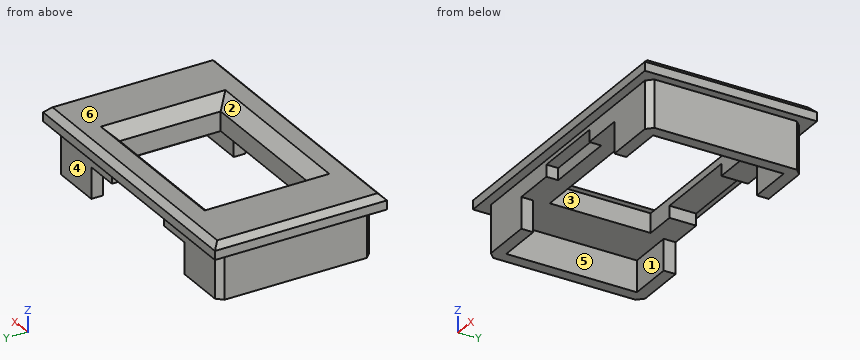
from build123d import *

# Parameters (mm, degrees)
SKETCH_W        = 45
SKETCH_H        = 26
PAD_DEPTH       = 8
SKETCH001_W     = 48
SKETCH001_H     = 29
PAD001_DEPTH    = 2.5
SKETCH002_W     = 25
SKETCH002_H     = 17
POCKET_DEPTH    = 10.501
SKETCH003_W     = 41
SKETCH003_H     = 22
POCKET001_DEPTH = 5.25
SKETCH004_W     = 26
SKETCH004_H     = 27.5
POCKET002_DEPTH = 5.251
SKETCH005_W     = 12
SKETCH005_H     = 2.5
POCKET003_DEPTH = 2
SKETCH006_W     = 14.5
SKETCH006_H     = 4.5
POCKET004_DEPTH = 2
CHAMFER_SIZE    = 1
CHAMFER001_SIZE = 2
CHAMFER002_SIZE = 1


with BuildPart() as part:
    # Sketch → Pad (new body)
    with BuildSketch(Plane.XY):
        Rectangle(SKETCH_W, SKETCH_H)
    extrude(amount=PAD_DEPTH)

    # Sketch001 (on Face6 of Pad) → Pad001 (join)
    with BuildSketch(Plane.XY.offset(8)):
        Rectangle(SKETCH001_W, SKETCH001_H)
    extrude(amount=PAD001_DEPTH)

    # Sketch002 (on Face5 of Pad001) → Pocket (cut, through all)
    with BuildSketch(Plane.XY.offset(10.5)):
        Rectangle(SKETCH002_W, SKETCH002_H)
    extrude(amount=-POCKET_DEPTH, mode=Mode.SUBTRACT)

    # Sketch003 (on Face15 of Pocket) → Pocket001 (cut)
    with BuildSketch(Plane(origin=(0, 0, 0), x_dir=(1, 0, 0), z_dir=(0, 0, -1))):
        Rectangle(SKETCH003_W, SKETCH003_H)
    extrude(amount=-POCKET001_DEPTH, mode=Mode.SUBTRACT)

    # Sketch004 (on Face16 of Pocket001) → Pocket002 (cut, through all)
    with BuildSketch(Plane(origin=(0, 0, 5.25), x_dir=(1, 0, 0), z_dir=(0, 0, -1))):
        Rectangle(SKETCH004_W, SKETCH004_H)
    extrude(amount=POCKET002_DEPTH, mode=Mode.SUBTRACT)

    # Sketch005 (on Face17 of Pocket002) → Pocket003 (cut)
    with BuildSketch(Plane(origin=(0, 0, 5.25), x_dir=(1, 0, 0), z_dir=(0, 0, -1))):
        with Locations((0, 12.25)):
            Rectangle(SKETCH005_W, SKETCH005_H)
    extrude(amount=-POCKET003_DEPTH, mode=Mode.SUBTRACT)

    # Sketch006 (on Face27 of Pocket003) → Pocket004 (cut)
    with BuildSketch(Plane(origin=(0, 0, 5.25), x_dir=(1, 0, 0), z_dir=(0, 0, -1))):
        with Locations((0, -10.75)):
            Rectangle(SKETCH006_W, SKETCH006_H)
    extrude(amount=-POCKET004_DEPTH, mode=Mode.SUBTRACT)

    # Chamfer
    chamfer_edges = [part.edges().sort_by_distance(p)[0] for p in [
        (24, 0, 10.5),
        (0, -14.5, 10.5),
        (0, 14.5, 10.5),
        (-24, 0, 10.5),
    ]]
    chamfer(chamfer_edges, length=CHAMFER_SIZE)

    # Chamfer001
    chamfer001_edges = [part.edges().sort_by_distance(p)[0] for p in [
        (0, 8.5, 10.5),
        (-12.5, 0, 10.5),
        (0, -8.5, 10.5),
        (12.5, 0, 10.5),
    ]]
    chamfer(chamfer001_edges, length=CHAMFER001_SIZE)

    # Chamfer002
    chamfer002_edges = [part.edges().sort_by_distance(p)[0] for p in [
        (-22.5, 13, 4),
        (-22.5, -13, 4),
        (22.5, 13, 4),
        (22.5, -13, 4),
    ]]
    chamfer(chamfer002_edges, length=CHAMFER002_SIZE)


solid = part.part
The model under review builds one solid part; all positions refer to its coordinate system, in mm. Face numbers are marked on the shaded views. A direction names the side the tool comes from. Round coordinates to 2 decimals unless told otherwise and drop trailing zeros. Write each loop counter-clockwise with the first axis right and the second up, starting at its lowest first coordinate (ties: lowest second). Pieces come first, ordered by that corner, then holes. Notation, with made-up numbers: (23, 31.25) - (37, 31.25) arc R10 ccw to (37, 48.25) - close; hole circle Ø6 at (83.5, 1.25). An arc over 180 degrees is marked (long way). One line per item, written item: value. Start each with the question number.
1. Consider section C-C on y = 7. Write out the cut boundary in (x, z), and give its area (4 significant figures).
2. Consider section B-B on x = -2. Write out the cut boundary in (y, z), and give its area (4 significant figures).
3. To check wall thickness, follow L1, parallel to X at y = 5.5, z = 5; L2, parallel to X at y = 3.5, z = 9; L3, parallel to Y at x = 8, z = 7. State the ranges of each line that lie inside material, in increasing order. Write a range as from..to.
4. Clearance check with flat-ended pins moving along their axes: P1, Ø1, axis at y = 11, z = 6.5, coming from the +X side; P2, Ø4, axis at x = 18.5, z = 1.5, coming from the -Y side; P3, Ø1.6, axis at x = -4.5, z = 6.5, coming from the +Y side; P4, Ø6, axis at x = 11, y = 9, coming from the -Z side. State where each tip first meets the part, or that it passes through.
5. Consider section A-A on z = 2.75. Write out the cut boundary in (x, y), and give its area (3 significant figures).
6. The part is to be moulded in two halves that separate along Y. For the marked faces 4, 5 and 6, say which applies: released by +Y, released by -Y, zero draft, split by the parting line, or undercut.
7. Consider section D-D on z = 9. Write out the cut boundary in (x, y), and give its area (3 significant figures).
8. Machinability: for the marked faces 1, 2 and 3, which of the approach directions +Z, -Z, +X, -X, +Y, -Y give a long, thin tool a straight path to every point of the face, cutting with its end or side? Answer none if there is none.
Checks:
1. outline: (-24, 8) - (-22.5, 8) - (-22.5, 0) - (-20.5, 0) - (-20.5, 5.25) - (-12.5, 5.25) - (-12.5, 8.5) - (-14.5, 10.5) - (-23, 10.5) - (-24, 9.5) - close; (12.5, 5.25) - (20.5, 5.25) - (20.5, 0) - (22.5, 0) - (22.5, 8) - (24, 8) - (24, 9.5) - (23, 10.5) - (14.5, 10.5) - (12.5, 8.5) - close
1. area: 128.5 mm^2
2. outline: (-14.5, 8) - (-13, 8) - (-13, 7.25) - (-11, 7.25) - (-11, 5.25) - (-8.5, 5.25) - (-8.5, 8.5) - (-10.5, 10.5) - (-13.5, 10.5) - (-14.5, 9.5) - close; (8.5, 7.25) - (13, 7.25) - (13, 8) - (14.5, 8) - (14.5, 9.5) - (13.5, 10.5) - (10.5, 10.5) - (8.5, 8.5) - close
2. area: 36.75 mm^2
3. L1: x = -22.5..-20.5, 20.5..22.5
3. L2: x = -24..-13, 13..24
3. L3: y = -13..-8.5, 8.5..13
4. P1: stops at x = 22.5
4. P2: stops at y = -13
4. P3: stops at y = 13
4. P4: stops at z = 0
5. outline: (-22.5, -12) - (-21.5, -13) - (-13, -13) - (-13, -11) - (-20.5, -11) - (-20.5, 11) - (-13, 11) - (-13, 13) - (-21.5, 13) - (-22.5, 12) - close; (13, -13) - (21.5, -13) - (22.5, -12) - (22.5, 12) - (21.5, 13) - (13, 13) - (13, 11) - (20.5, 11) - (20.5, -11) - (13, -11) - close
5. area: 162 mm^2
6. face 4: released by +Y
6. face 5: undercut
6. face 6: zero draft
7. outline: (-24, -14.5) - (24, -14.5) - (24, 14.5) - (-24, 14.5) - close; hole (-13, -9) - (13, -9) - (13, 9) - (-13, 9) - close
7. area: 924 mm^2
8. face 1: -Z
8. face 2: +Z
8. face 3: +Z, -Z
